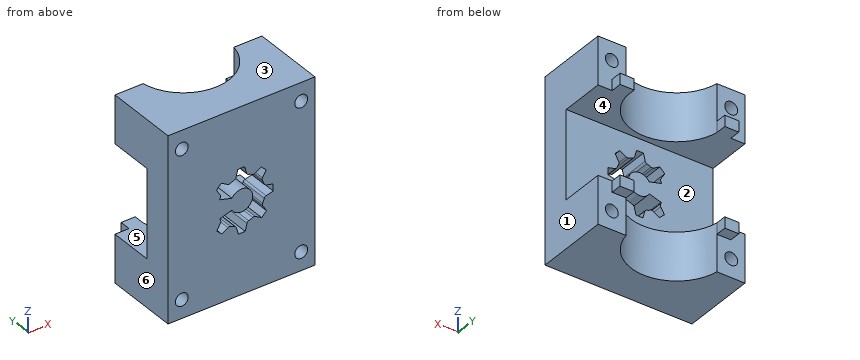
```python
from build123d import *

# Parameters (mm, degrees)
CROQUIS1_W              = 40
CROQUIS1_H              = 50
SALIENTE_EXTRUIR1_DEPTH = 20
CROQUIS2_R              = 12.5
CORTAR_EXTRUIR1_DEPTH   = 51
CROQUIS3_R              = 1.75
CORTAR_EXTRUIR2_DEPTH   = 21
CORTAR_EXTRUIR3_DEPTH   = 41
CROQUIS5_W              = 3.830518661
CROQUIS5_H              = 3
SALIENTE_EXTRUIR3_DEPTH = 3
CORTAR_EXTRUIR5_DEPTH   = 24


with BuildPart() as part:
    # Croquis1 → Saliente-Extruir1 (new body)
    with BuildSketch(Plane(origin=(0, 0, 0), x_dir=(1, 0, 0), z_dir=(0, 1, 0))):
        with Locations((20, 25)):
            Rectangle(CROQUIS1_W, CROQUIS1_H)
    extrude(amount=SALIENTE_EXTRUIR1_DEPTH)

    # Croquis2 → Cortar-Extruir1 (cut, through all)
    with BuildSketch(Plane.XY):
        with Locations((20, 22)):
            Circle(CROQUIS2_R)
    extrude(amount=-CORTAR_EXTRUIR1_DEPTH, mode=Mode.SUBTRACT)

    # Croquis3 → Cortar-Extruir2 (cut, through all)
    with BuildSketch(Plane(origin=(0, 20, 0), x_dir=(1, 0, 0), z_dir=(0, 1, 0))):
        with Locations((3.75, 45)):
            Circle(CROQUIS3_R)
        with Locations((36.25, 45)):
            Circle(CROQUIS3_R)
        with Locations((36.25, 5)):
            Circle(CROQUIS3_R)
        with Locations((3.75, 5)):
            Circle(CROQUIS3_R)
    extrude(amount=-CORTAR_EXTRUIR2_DEPTH, mode=Mode.SUBTRACT)

    # Croquis4 → Cortar-Extruir3 (cut, through all)
    with BuildSketch(Plane(origin=(40, 0, 0), x_dir=(0, 0, -1), z_dir=(1, 0, 0))):
        Polygon((25, 20), (37, 20), (37, 8), (13, 8), (13, 20), align=None)
    extrude(amount=-CORTAR_EXTRUIR3_DEPTH, mode=Mode.SUBTRACT)

    # Croquis5 → Saliente-Extruir3 (add)
    with BuildSketch(Plane(origin=(0, 20, 0), x_dir=(1, 0, 0), z_dir=(0, 1, 0))):
        with Locations((5.745777991, 38.5)):
            Rectangle(CROQUIS5_W, CROQUIS5_H)
        with Locations((34.25422201, 38.5)):
            Rectangle(CROQUIS5_W, CROQUIS5_H)
        with Locations((34.25422201, 11.5)):
            Rectangle(CROQUIS5_W, CROQUIS5_H)
        with Locations((5.745777991, 11.5)):
            Rectangle(CROQUIS5_W, CROQUIS5_H)
    extrude(amount=SALIENTE_EXTRUIR3_DEPTH)

    # Croquis6 → Cortar-Extruir5 (cut, through all)
    with BuildSketch(Plane.XZ):
        with BuildLine():
            Line((13.188139939, -19.615331161), (14.501537669, -18.279657152))
            Line((14.501537669, -18.279657152), (16.224863288, -19.28260268))
            ThreePointArc((16.224863288, -19.28260268), (16.575067996, -19.380217097), (16.928320792, -19.294284721))
            ThreePointArc((16.928320792, -19.294284721), (17.469957789, -19.034324312), (18.033343063, -18.825644933))
            ThreePointArc((18.033343063, -18.825644933), (18.340671144, -18.631425053), (18.513928995, -18.31181024))
            Line((18.513928995, -18.31181024), (18.990823409, -16.375751708))
            Line((18.990823409, -16.375751708), (20.864, -16.36))
            Line((20.864, -16.36), (21.373385647, -18.287764816))
            ThreePointArc((21.373385647, -18.287764816), (21.551993955, -18.604420755), (21.862544768, -18.793444837))
            ThreePointArc((21.862544768, -18.793444837), (22.429359729, -18.992620263), (22.975291881, -19.243435206))
            ThreePointArc((22.975291881, -19.243435206), (23.329939845, -19.323414782), (23.678453448, -19.219924782))
            Line((23.678453448, -19.219924782), (25.384668839, -18.188139939))
            Line((25.384668839, -18.188139939), (26.720342848, -19.501537669))
            Line((26.720342848, -19.501537669), (25.71739732, -21.224863288))
            ThreePointArc((25.71739732, -21.224863288), (25.619782903, -21.575067996), (25.705715279, -21.928320792))
            ThreePointArc((25.705715279, -21.928320792), (25.965675688, -22.469957789), (26.174355067, -23.033343063))
            ThreePointArc((26.174355067, -23.033343063), (26.368574947, -23.340671144), (26.68818976, -23.513928995))
            Line((26.68818976, -23.513928995), (28.624248292, -23.990823409))
            Line((28.624248292, -23.990823409), (28.64, -25.864))
            Line((28.64, -25.864), (26.712235184, -26.373385647))
            ThreePointArc((26.712235184, -26.373385647), (26.395579245, -26.551993955), (26.206555163, -26.862544768))
            ThreePointArc((26.206555163, -26.862544768), (26.007379737, -27.429359729), (25.756564794, -27.975291881))
            ThreePointArc((25.756564794, -27.975291881), (25.676585218, -28.329939845), (25.780075218, -28.678453448))
            Line((25.780075218, -28.678453448), (26.811860061, -30.384668839))
            Line((26.811860061, -30.384668839), (25.498462331, -31.720342848))
            Line((25.498462331, -31.720342848), (23.775136712, -30.71739732))
            ThreePointArc((23.775136712, -30.71739732), (23.424932004, -30.619782903), (23.071679208, -30.705715279))
            ThreePointArc((23.071679208, -30.705715279), (22.530042211, -30.965675688), (21.966656937, -31.174355067))
            ThreePointArc((21.966656937, -31.174355067), (21.659328856, -31.368574947), (21.486071005, -31.68818976))
            Line((21.486071005, -31.68818976), (21.009176591, -33.624248292))
            Line((21.009176591, -33.624248292), (19.136, -33.64))
            Line((19.136, -33.64), (18.626614353, -31.712235184))
            ThreePointArc((18.626614353, -31.712235184), (18.448006045, -31.395579245), (18.137455232, -31.206555163))
            ThreePointArc((18.137455232, -31.206555163), (17.570640271, -31.007379737), (17.024708119, -30.756564794))
            ThreePointArc((17.024708119, -30.756564794), (16.670060155, -30.676585218), (16.321546552, -30.780075218))
            Line((16.321546552, -30.780075218), (14.615331161, -31.811860061))
            Line((14.615331161, -31.811860061), (13.279657152, -30.498462331))
            Line((13.279657152, -30.498462331), (14.28260268, -28.775136712))
            ThreePointArc((14.28260268, -28.775136712), (14.380217097, -28.424932004), (14.294284721, -28.071679208))
            ThreePointArc((14.294284721, -28.071679208), (14.208247472, -27.906200724), (14.127008205, -27.738314697))
            ThreePointArc((14.127008205, -27.738314697), (14.125953752, -27.626452127), (14.209575503, -27.552143653))
            Line((14.209575503, -27.552143653), (17.384042323, -26.571445385))
            ThreePointArc((17.384042323, -26.571445385), (23.05159058, -25.021681648), (17.406635637, -23.391542216))
            Line((17.406635637, -23.391542216), (14.170602247, -22.54767412))
            ThreePointArc((14.170602247, -22.54767412), (14.082937198, -22.475491969), (14.08129489, -22.361945826))
            ThreePointArc((14.08129489, -22.361945826), (14.159930296, -22.19215637), (14.243435206, -22.024708119))
            ThreePointArc((14.243435206, -22.024708119), (14.323414782, -21.670060155), (14.219924782, -21.321546552))
            Line((14.219924782, -21.321546552), (13.188139939, -19.615331161))
        make_face()
    extrude(amount=-CORTAR_EXTRUIR5_DEPTH, mode=Mode.SUBTRACT)


solid = part.part
```
Design review of the part built by this model. Coordinates are the model's own, in mm. Face numbers are marked on the shaded views. A direction names the side the tool comes from. Coordinates: 2 decimals unless noted, no trailing zeros. Order: outer loops, then holes, each group sorted by start corner. A loop starts at its lowest first (then second) coordinate and runs counter-clockwise, first axis right, second up. Notation, with made-up numbers: (26.5, 64) -> (31.5, 64) arc R22 cw to (31.5, 96) -> close; hole circle Ø7 at (52.25, 23). An arc over 180 degrees is marked (long way). One line per item, written item: value. Start each with the question number.
Q1. Mouldability with a two-part tool opening along Z and no side actions: class the marked faces 1, 2, 3 and 4 as pulls with the +Z half, pulls with the -Z half, needs draft (parallel to the pull), parting line crosses it, or undercut.
Q2. Insertion check: pin 1 Ø12 at (x, y) = (22, 12.5) entering from -Z; pin 2 Ø2.5 at (x, z) = (35.5, -4) entering from +Y; pin 3 Ø1.5 at (x, y) = (6, 21) entering from +Z; pin 4 Ø12 at (x, z) = (20, -20.5) entering from +Y. Each pin has a flat end and moves straight along its axis. Give the tip position at first contact, or say it passes through.
Q3. Take a section at D-D, the plane x = 9. State the section outline as (y, z) points, then the cut area to 3 significant figures.
Q4. Take a section at B-B, the plane y = 18.25. State the section outline as (x, z) points.
Q5. Take a section at A-A, the plane z = -45. State the section outline as (x, y) points.
Q6. Tool access review of the marked faces 5 and 6: name each direction out of +Z, -Z, +X, -X, +Y, -Y from which nothing blocks a thin tool from reaching the whole face with its end or side.
Q7. Take a section at C-C, the plane z = -38.5. State the section outline as (x, y) points, then the cut area to 3 significant figures.
Q8. For probe 1 along Z at (x, y) = (36.25, 11); probe 2 along X at (y, z) = (6, -45); probe 3 along Z at (x, y) = (6, 21.75), list the stretches that pass through material, from the lowest coordinate up.
Values follow:
1. face 1: needs draft
1. face 2: undercut
1. face 3: pulls with the +Z half
1. face 4: undercut
2. pin 1: stops at z = -50
2. pin 2: stops at y = 20
2. pin 3: stops at z = -10
2. pin 4: stops at y = 8
3. outline: (0, -50) -> (16.06, -50) -> (16.06, -37) -> (8, -37) -> (8, -13) -> (16.06, -13) -> (16.06, 0) -> (0, 0) -> close
3. area: 610 mm2
4. outline: (0, -50) -> (8.08, -50) -> (8.08, -37) -> (0, -37) -> close; (0, -13) -> (8.08, -13) -> (8.08, 0) -> (0, 0) -> close; (31.92, -50) -> (40, -50) -> (40, -37) -> (31.92, -37) -> close; (31.92, -13) -> (40, -13) -> (40, 0) -> (31.92, 0) -> close; hole circle Ø3.5 at (3.75, -45); hole circle Ø3.5 at (3.75, -5); hole circle Ø3.5 at (36.25, -45); hole circle Ø3.5 at (36.25, -5)
5. outline: (0, 0) -> (2, 0) -> (2, 20) -> (0, 20) -> close; (5.5, 0) -> (34.5, 0) -> (34.5, 20) -> (32.34, 20) arc R12.5 cw to (7.66, 20) -> (5.5, 20) -> close; (38, 0) -> (40, 0) -> (40, 20) -> (38, 20) -> close
6. face 5: +X, -X, +Y
6. face 6: +Z, -Z, -X, +Y, -Y
7. outline: (0, 0) -> (40, 0) -> (40, 20) -> (36.17, 20) -> (36.17, 23) -> (32.34, 23) -> (32.34, 20) arc R12.5 cw to (7.66, 20) -> (7.66, 23) -> (3.83, 23) -> (3.83, 20) -> (0, 20) -> close
7. area: 627 mm2
8. probe 1: z = -50 to -46.75, -43.25 to -37, -13 to -6.75, -3.25 to 0
8. probe 2: x = 0 to 2, 5.5 to 34.5, 38 to 40
8. probe 3: z = -40 to -37, -13 to -10
